Design review of the part built by this model. Coordinates are the model's own, in mm. A direction names the side the tool comes from. Coordinates: 2 decimals unless noted, no trailing zeros. Write each loop counter-clockwise with the first axis right and the second up, starting at its lowest first coordinate (ties: lowest second). Pieces come first, ordered by that corner, then holes. Notation, with made-up numbers: (-12, 8) -> (14, 8) arc R20 ccw to (14, 35) -> close; hole circle Ø5 at (-23, -15.75). An arc over 180 degrees is marked (long way). Write item = value, one per line. Start each with the question number.
Autodesk Inventor part; units mm, degrees
ref_plane "YZ Plane" through (0, 0, 0) normal (1, 0, 0) x (0, 1, 0)
ref_plane "XZ Plane" through (0, 0, 0) normal (0, 1, 0) x (-1, 0, 0)
ref_plane "XY Plane" through (0, 0, 0) normal (0, 0, 1) x (1, 0, 0)
sketch "Sketch1" plane through (0, 0, 0) normal (0, 0, 1) x (1, 0, 0)
  line L0 (-1, -2.5) -> (1, -2.5)
  line L1 (1, -2.5) -> (1, 2.5)
  line L2 (1, 2.5) -> (-1, 2.5)
  line L3 (-1, 2.5) -> (-1, -2.5)
  line L4 (-1, -2.5) -> (1, 2.5) construction
  line L5 (1, -2.5) -> (-1, 2.5) construction
  line L6 (-2, -3.5) -> (2, -3.5)
  line L7 (2, -3.5) -> (2, 3.5)
  line L8 (2, 3.5) -> (-2, 3.5)
  line L9 (-2, 3.5) -> (-2, -3.5)
  line L10 (-2, -3.5) -> (2, 3.5) construction
  line L11 (2, -3.5) -> (-2, 3.5) construction
  point P0 (0, 0)
  point P1 (0, 0)
  dimension "d5" = 2
  dimension "d6" = 5
  dimension "d7" = 4
  dimension "d8" = 7
extrude "Extrusion1" add sketch "Sketch1" along normal blind 4.5
fillet "Fillet1" radius 2 4 edges at (2, 3.5, 2.25) (-2, 3.5, 2.25) (2, -3.5, 2.25) (-2, -3.5, 2.25)
fillet "Fillet2" radius 0.5 4 edges at (-1, 2.5, 2.25) (1, 2.5, 2.25) (-1, -2.5, 2.25) (1, -2.5, 2.25)
properties part number "COILS" material "Copper"
(1) Take a section at A-A, the plane y = -0.75. State the section outline as (x, z) points, then the cut area to 3 significant figures.
(2) For faces 4 (the face through (2, 0, 2)), 5 (the face through (1, 0, 2)), list the 3-axis set-ups (+Z, -Z, +X, -X, +Y, -Y) from which the entire face can be reached by the end or side of a thin tool; tool diameter is ignored.
(3) Take a section at B-B, the plane x = 0.9. State the section outline as (y, z) points.
(4) For line 1 (X direction, y = 1.5, z = 3.7); line 2 (Y direction, x = 0.1, z = 1.45); line 3 (Y direction, x = -0.7, z = 2.6), list the stretches that pass through material, from the lowest coordinate up.
(5) Mouldability with a two-part tool opening along X and no side actions: class faces 1 (the face through (0, -2.5, 2)), 2 (the face through (-2, 0, 2)), 3 (the face through (1.43, 2.9, 2.28)) as pulls with the +X half, pulls with the -X half, needs draft (parallel to the pull), parting line crosses it, or undercut.
(6) Take a section at D-D, the plane x = -1.65. State the section outline as (y, z) points, then the cut area to 3 significant figures.
Report:
q1.outline = (-2, 0) -> (-1, 0) -> (-1, 4.5) -> (-2, 4.5) -> close; (1, 0) -> (2, 0) -> (2, 4.5) -> (1, 4.5) -> close
q1.area = 9.00 mm2
q2.face_4 = +Z, -Z, +X, +Y, -Y
q2.face_5 = +Z, -Z
q3.outline = (-3.29, 0) -> (-2.3, 0) -> (-2.3, 4.5) -> (-3.29, 4.5) -> close; (2.3, 0) -> (3.29, 0) -> (3.29, 4.5) -> (2.3, 4.5) -> close
q4.line_1 = -2 to -1, 1 to 2
q4.line_2 = -3.5 to -2.5, 2.5 to 3.5
q4.line_3 = -3.37 to -2.46, 2.46 to 3.37
q5.face_1 = undercut
q5.face_2 = pulls with the -X half
q5.face_3 = pulls with the +X half
q6.outline = (-2.63, 0) -> (2.63, 0) -> (2.63, 4.5) -> (-2.63, 4.5) -> close
q6.area = 23.7 mm2
